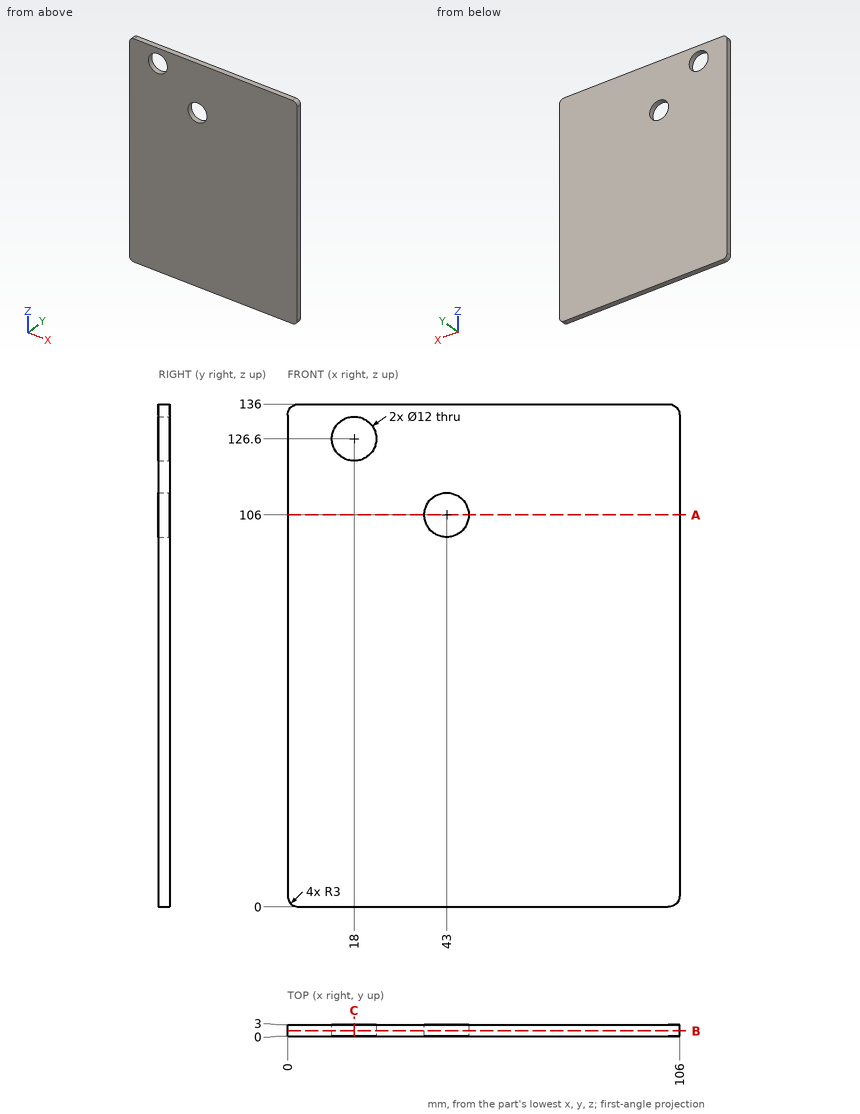
Input: dimensioned drawing with shaded views. Units: mm. Origin: part minimum x, y, z. Give positions to 0.01 mm unless a question says otherwise; leave off trailing zeros. Order: outer loops, then holes, each group sorted by start corner. A loop starts at its lowest first (then second) coordinate and runs counter-clockwise, first axis right, second up.
(1) Section query B-B (y = 1.4). Return the cut outline in (x, z), plus the area to 3 significant figures.
(2) Contact query for a flat-ended pin moving along its axis: P1, Ø11, axis at x = 18, z = 126.6, coming from the -Y side. Output: stop coordinate, or through.
(3) Material intervals for line 1 along Z through (x, y) = (43, 2.4); line 2 along X through (y, z) = (1.55, 106); line 3 along X through (y, z) = (2.35, 126.6), sorted ascending.
(4) Section query A-A (z = 106). Return the cut outline in (x, y).
(5) Section query C-C (x = 18). Return the cut outline in (y, z).
Outcome:
1. outline: (0, 3) arc R3 ccw to (3, 0) - (103, 0) arc R3 ccw to (106, 3) - (106, 133) arc R3 ccw to (103, 136) - (3, 136) arc R3 ccw to (0, 133) - close; hole circle Ø12 at (18, 126.6); hole circle Ø12 at (43, 106)
1. area: 14,200 mm2
2. P1: passes through
3. line 1: z = 0 to 100, 112 to 136
3. line 2: x = 0 to 37, 49 to 106
3. line 3: x = 0 to 12, 24 to 106
4. outline: (0, 0) - (37, 0) - (37, 3) - (0, 3) - close; (49, 0) - (106, 0) - (106, 3) - (49, 3) - close
5. outline: (0, 0) - (3, 0) - (3, 120.6) - (0, 120.6) - close; (0, 132.6) - (3, 132.6) - (3, 136) - (0, 136) - close
